Geometry check sheet. Reference: the model listing, model coordinates, mm. A direction names the side the tool comes from. Give positions to 0.01 mm unless a question says otherwise; leave off trailing zeros. Write each loop counter-clockwise with the first axis right and the second up, starting at its lowest first coordinate (ties: lowest second). Pieces come first, ordered by that corner, then holes. Notation, with made-up numbers: (32.25, 49) -> (85.25, 49) arc R6 ccw to (85.25, 60) -> close; hole circle Ø4 at (25.25, 39). An arc over 180 degrees is marked (long way). One line per item, written item: value.
from build123d import *

# Parameters (mm, degrees)
CYLINDER031_R          = 2.5
CYLINDER031_DEPTH      = 14
CYLINDER030_R          = 2.5
CYLINDER030_DEPTH      = 14
BOX012_W               = 134
BOX012_H               = 152
BOX012_DEPTH           = 11
BOX012_ROLL_ANGLE      = 25.000043
BOX012_PLACEMENT_ANGLE = 180
BOX011_W               = 10
BOX011_H               = 10
BOX011_DEPTH           = 10
BOX010_W               = 140
BOX010_H               = 162
BOX010_DEPTH           = 4
BOX010_ROLL_ANGLE      = 25.000043
BOX010_PLACEMENT_ANGLE = 180
CYLINDER004_W          = 5.4
CYLINDER004_H          = 10
CYLINDER004_ANGLE      = 90
BOX009_W               = 10
BOX009_H               = 6
BOX009_DEPTH           = 25
BOX009_PLACEMENT_ANGLE = 65
BOX008_W               = 10
BOX008_H               = 6
BOX008_DEPTH           = 31.23
BOX007_W               = 10
BOX007_H               = 2
BOX007_DEPTH           = 165
BOX002_W               = 140
BOX002_H               = 162
BOX002_DEPTH           = 4
BOX002_ROLL_ANGLE      = 25.000043
BOX002_PLACEMENT_ANGLE = 180
CYLINDER001_W          = 18
CYLINDER001_H          = 10
CYLINDER001_ANGLE      = 65
CYLINDER_W             = 18
CYLINDER_H             = 10
CYLINDER_ANGLE         = 65
BOX004_W               = 10
BOX004_H               = 6
BOX004_DEPTH           = 81
BOX006_W               = 10
BOX006_H               = 6
BOX006_DEPTH           = 20
CYLINDER003_W          = 18
CYLINDER003_H          = 10
CYLINDER003_ANGLE      = 25
CYLINDER002_W          = 18
CYLINDER002_H          = 10
CYLINDER002_ANGLE      = 25
BOX043_W               = 10
BOX043_H               = 109
BOX043_DEPTH           = 4


with BuildPart() as m4s008:
    # Cylinder031 → Cylinder031 (new body)
    with BuildSketch(Plane(origin=(105, 264, 0), x_dir=(1, 0, 0), z_dir=(0, 0, 1))):
        Circle(CYLINDER031_R)
    extrude(amount=CYLINDER031_DEPTH)


with BuildPart() as fusion015:
    # Cylinder030 → Cylinder030 (new body)
    with BuildSketch(Plane(origin=(105, 144.5, 0), x_dir=(1, 0, 0), z_dir=(0, 0, 1))):
        Circle(CYLINDER030_R)
    extrude(amount=CYLINDER030_DEPTH)

    # Fusion015: union m4s008
    add(m4s008.part)


with BuildPart() as solar_panelcut:
    # Box012 → Box012 (new body)
    with BuildSketch(Plane.XY):
        with Locations((67, 76)):
            Rectangle(BOX012_W, BOX012_H)
    extrude(amount=BOX012_DEPTH)


with BuildPart() as solar_panelcut_1:
    # Box012 roll: moved
    add(solar_panelcut.part.rotate(Axis((0, 0, 0), (1, 0, 0)), BOX012_ROLL_ANGLE))


with BuildPart() as solar_panelcut_2:
    # Box012 placement: moved
    add(solar_panelcut_1.part.moved(Location((175, 279.468463, 10.113095))).rotate(Axis((175, 279.468463, 10.113095), (0, 0, 1)), BOX012_PLACEMENT_ANGLE))


with BuildPart() as cube:
    # Box011 → Box011 (new body)
    with BuildSketch(Plane(origin=(100, 289.23, 0), x_dir=(1, 0, 0), z_dir=(0, 0, 1))):
        with Locations((5, 5)):
            Rectangle(BOX011_W, BOX011_H)
    extrude(amount=BOX011_DEPTH)


with BuildPart() as solar_panel004:
    # Box010 → Box010 (new body)
    with BuildSketch(Plane.XY):
        with Locations((70, 81)):
            Rectangle(BOX010_W, BOX010_H)
    extrude(amount=BOX010_DEPTH)


with BuildPart() as solar_panel004_1:
    # Box010 roll: moved
    add(solar_panel004.part.rotate(Axis((0, 0, 0), (1, 0, 0)), BOX010_ROLL_ANGLE))


with BuildPart() as solar_panel004_2:
    # Box010 placement: moved
    add(solar_panel004_1.part.moved(Location((175, 284, 8))).rotate(Axis((175, 284, 8), (0, 0, 1)), BOX010_PLACEMENT_ANGLE))


with BuildPart() as cylinder004:
    # Cylinder004 → Cylinder004 (revolve)
    with BuildSketch(Plane(origin=(110, 283.83, 10), x_dir=(0, 0, 1), z_dir=(0, -1, 0))):
        with Locations((2.7, 5)):
            Rectangle(CYLINDER004_W, CYLINDER004_H)
    revolve(axis=Axis((110, 283.83, 10), (-1, 0, 0)), revolution_arc=CYLINDER004_ANGLE)


with BuildPart() as basesupport007:
    # Box009 → Box009 (new body)
    with BuildSketch(Plane.XY):
        with Locations((5, 3)):
            Rectangle(BOX009_W, BOX009_H)
    extrude(amount=BOX009_DEPTH)


with BuildPart() as basesupport007_1:
    # Box009 placement: moved
    add(basesupport007.part.moved(Location((100, 284.507102, 8.798097))).rotate(Axis((100, 284.507102, 8.798097), (1, 0, 0)), BOX009_PLACEMENT_ANGLE))


with BuildPart() as basesupport006:
    # Box008 → Box008 (new body)
    with BuildSketch(Plane(origin=(100, 258, 10), x_dir=(1, 0, 0), z_dir=(0, 1, 0))):
        with Locations((5, 3)):
            Rectangle(BOX008_W, BOX008_H)
    extrude(amount=BOX008_DEPTH)


with BuildPart() as basesupport005:
    # Box007 → Box007 (new body)
    with BuildSketch(Plane(origin=(100, 131, 6), x_dir=(1, 0, 0), z_dir=(0, 1, 0))):
        with Locations((5, 1)):
            Rectangle(BOX007_W, BOX007_H)
    extrude(amount=BOX007_DEPTH)


with BuildPart() as solar_panel001:
    # Box002 → Box002 (new body)
    with BuildSketch(Plane.XY):
        with Locations((70, 81)):
            Rectangle(BOX002_W, BOX002_H)
    extrude(amount=BOX002_DEPTH)


with BuildPart() as solar_panel001_1:
    # Box002 roll: moved
    add(solar_panel001.part.rotate(Axis((0, 0, 0), (1, 0, 0)), BOX002_ROLL_ANGLE))


with BuildPart() as solar_panel001_2:
    # Box002 placement: moved
    add(solar_panel001_1.part.moved(Location((175, 284, 8))).rotate(Axis((175, 284, 8), (0, 0, 1)), BOX002_PLACEMENT_ANGLE))


with BuildPart() as cylinder001:
    # Cylinder001 → Cylinder001 (revolve)
    with BuildSketch(Plane(origin=(101, 137, 72.5), x_dir=(0, 0, -1), z_dir=(0, -1, 0))):
        with Locations((9, 5)):
            Rectangle(CYLINDER001_W, CYLINDER001_H)
    revolve(axis=Axis((101, 137, 72.5), (1, 0, 0)), revolution_arc=CYLINDER001_ANGLE)


with BuildPart() as basesupport001:
    # Cylinder → Cylinder (revolve)
    with BuildSketch(Plane(origin=(101, 137, 85), x_dir=(0, 0, -1), z_dir=(0, -1, 0))):
        with Locations((9, 5)):
            Rectangle(CYLINDER_W, CYLINDER_H)
    revolve(axis=Axis((101, 137, 85), (1, 0, 0)), revolution_arc=CYLINDER_ANGLE)

    # Cut: cut Cylinder001
    add(cylinder001.part, mode=Mode.SUBTRACT)


with BuildPart() as basesupport001_1:
    # Cut placement: moved
    add(basesupport001.part.moved(Location((-1, 0, 0))))


with BuildPart() as basesupport003:
    # Box004 → Box004 (new body)
    with BuildSketch(Plane(origin=(100, 131, 4), x_dir=(1, 0, 0), z_dir=(0, 0, 1))):
        with Locations((5, 3)):
            Rectangle(BOX004_W, BOX004_H)
    extrude(amount=BOX004_DEPTH)

    # Fusion: union baseSupport001
    add(basesupport001_1.part)

    # Cut001: cut solar Panel001
    add(solar_panel001_2.part, mode=Mode.SUBTRACT)


with BuildPart() as basesupport004:
    # Box006 → Box006 (new body)
    with BuildSketch(Plane(origin=(100, 131, 10), x_dir=(1, 0, 0), z_dir=(0, 1, 0))):
        with Locations((5, 3)):
            Rectangle(BOX006_W, BOX006_H)
    extrude(amount=BOX006_DEPTH)


with BuildPart() as cylinder003:
    # Cylinder003 → Cylinder003 (revolve)
    with BuildSketch(Plane(origin=(110, 280.25, 6), x_dir=(0, -1, 0), z_dir=(0, 0, -1))):
        with Locations((9, 5)):
            Rectangle(CYLINDER003_W, CYLINDER003_H)
    revolve(axis=Axis((110, 280.25, 6), (-1, 0, 0)), revolution_arc=CYLINDER003_ANGLE)


with BuildPart() as obj1:
    # Cylinder002 → Cylinder002 (revolve)
    with BuildSketch(Plane(origin=(110, 288.25, 6), x_dir=(0, -1, 0), z_dir=(0, 0, -1))):
        with Locations((9, 5)):
            Rectangle(CYLINDER002_W, CYLINDER002_H)
    revolve(axis=Axis((110, 288.25, 6), (-1, 0, 0)), revolution_arc=CYLINDER002_ANGLE)

    # Cut002: cut Cylinder003
    add(cylinder003.part, mode=Mode.SUBTRACT)

    # Fusion001: union Cylinder004, baseSupport007, baseSupport006, baseSupport005, baseSupport003, baseSupport004
    add(cylinder004.part)
    add(basesupport007_1.part)
    add(basesupport006.part)
    add(basesupport005.part)
    add(basesupport003.part)
    add(basesupport004.part)

    # Cut003: cut solar Panel004
    add(solar_panel004_2.part, mode=Mode.SUBTRACT)

    # Cut004: cut Cube
    add(cube.part, mode=Mode.SUBTRACT)

    # Cut005: cut solar PanelCut
    add(solar_panelcut_2.part, mode=Mode.SUBTRACT)

    # Cut030: cut Fusion015
    add(fusion015.part, mode=Mode.SUBTRACT)


with BuildPart() as obj1_1:
    # Cut030 placement: moved
    add(obj1.part.moved(Location((-1, 0, 0))))


with BuildPart() as obj2:
    # Box043 → Box043 (new body)
    with BuildSketch(Plane(origin=(99, 150, 6), x_dir=(1, 0, 0), z_dir=(0, 0, 1))):
        with Locations((5, 54.5)):
            Rectangle(BOX043_W, BOX043_H)
    extrude(amount=BOX043_DEPTH)

    # Fusion029: union obj1
    add(obj1_1.part)


solid = obj2.part
1) Sectioned sample at C-C on y = 153.5. Record the cut outline in (x, z).
Verdict:
outline: (99, 4) -> (109, 4) -> (109, 10) -> (99, 10) -> close
2) Sectioned sample at A-A on y = 264. Record the cut outline in (x, z).
Verdict:
outline: (99, 4) -> (101.5, 4) -> (101.5, 10) -> (99, 10) -> close; (106.5, 4) -> (109, 4) -> (109, 10) -> (106.5, 10) -> close
3) Sectioned sample at D-D on z = 22.5. Record the cut outline in (x, y), plus the area to 3 significant figures.
Verdict:
outline: (99, 131) -> (109, 131) -> (109, 137) -> (99, 137) -> close
area: 60.0 mm^2
4) Scan lines: probe 1 along X at (y, z) = (264, 5.75); probe 2 along Y at (x, z) = (104, 6.6); probe 3 along Z at (x, y) = (106.5, 212.5). Record each from-to range of solid material in increasing order.
Verdict:
probe 1: 99 to 101.5, 106.5 to 109
probe 2: 131 to 142, 147 to 261.5, 266.5 to 289.23
probe 3: 4 to 10
5) Depth check by flat-ended pin: pin 1 Ø2 at (x, y) = (103.5, 156.5) entering from +Z; pin 2 Ø4.5 at (x, y) = (104, 264) entering from -Z; pin 3 Ø3 at (x, z) = (100, 30) entering from +Y. Enter the tip coordinate at first touch or a pass-through.
Verdict:
pin 1: z = 10
pin 2: through
pin 3: y = 137
6) Mould release check, pull along Z, two halves, no side actions. Record for faces 1 (the flat face through (104.07, 138.01, 78.25)), 2 (the cylindrical face through (103.93, 287.91, 13.54)), 3 (the cylindrical face through (105.34, 146.61, 6.96)): released by +Z, released by -Z, zero draft, split by the parting line, or undercut.
Verdict:
face 1: undercut
face 2: released by +Z
face 3: zero draft
7) Tool access check on faces 4 (the flat face through (104.07, 283.39, 12.7)), 5 (the cylindrical face through (103.93, 271.284, 12.012)), 6 (the flat face through (104.07, 144.16, 79.61)), 7 (the flat face through (104, 209, 4)). Record the directions out of +Z, -Z, +X, -X, +Y, -Y that give a thin tool (end or side, any length) a straight path to the whole face; none if there is none.
Verdict:
face 4: +X, -X
face 5: +Z, +X, -X
face 6: +X, -X, +Y
face 7: -Z, +X, -X, +Y, -Y
8) Sectioned sample at B-B on x = 104. Give the number of separate pieces and of enclosed holes in the cut face, plus the area to 3 significant figures.
Verdict:
separate pieces: 3
enclosed holes: 0
area: 1,450 mm^2
